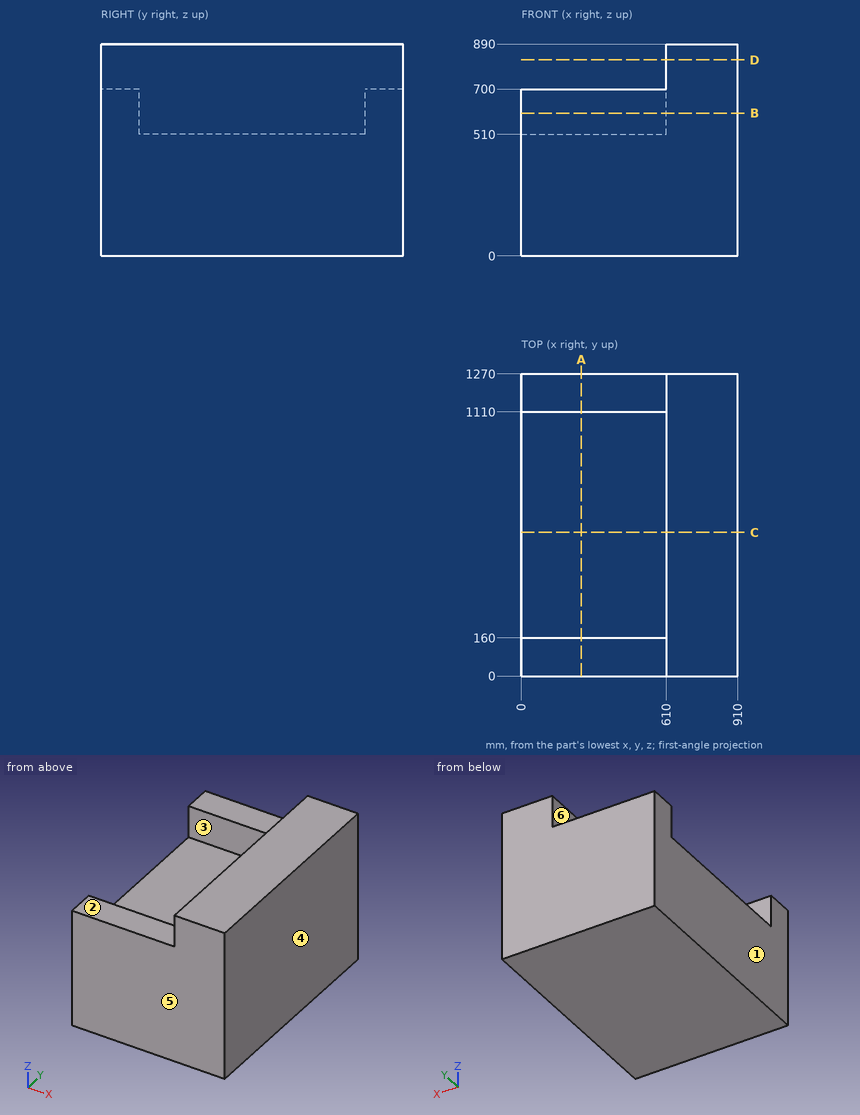
The figure shows three views and two pictorial views of one solid part (mm, origin at its lowest corner). Answer the questions. A direction names the side the tool comes from. Round coordinates to 2 decimals unless told otherwise and drop trailing zeros. Order: outer loops, then holes, each group sorted by start corner. A loop starts at its lowest first (then second) coordinate and runs counter-clockwise, first axis right, second up. Notation, with made-up numbers: (-13, -4.75) -> (14, -4.75) arc R10 cw to (14, -0.75) -> close; hole circle Ø7 at (82.5, 89). An arc over 180 degrees is marked (long way). One line per item, written item: value.
Item 1: Find section D-D, the plane z = 823. Give the vertices of the cut face in (x, y), then the cut area to 3 significant figures.
Taken from the geometry:
outline: (610, 0) -> (910, 0) -> (910, 1270) -> (610, 1270) -> close
area: 381,000 mm2
Item 2: For the marked faces 1, 2 and 3, determine the directions among +Z, -Z, +X, -X, +Y, -Y from which every point of the face is accessible in a straight line to the end or side of a thin tool.
Taken from the geometry:
face 1: +Z, -Z, -X, +Y, -Y
face 2: +Z, -X, +Y, -Y
face 3: +Z, -X
Item 3: Given P1, Ø10, axis at y = 164.5, z = 800.5, coming from the -X side, flat-ended and moving along its own axis, determine where the tip first touches the part or whether it passes through.
Taken from the geometry:
P1: stops at x = 610
Item 4: For a pull along Y with two mould halves and no side action, classify the marked faces 4, 5 and 6 as released by +Y, released by -Y, zero draft, split by the parting line, or undercut.
Taken from the geometry:
face 4: zero draft
face 5: released by -Y
face 6: undercut
Item 5: Find section A-A, the plane x = 252. Give the vertices of the cut face in (y, z), then the cut area to 4 significant figures.
Taken from the geometry:
outline: (0, 0) -> (1270, 0) -> (1270, 700) -> (1110, 700) -> (1110, 510) -> (160, 510) -> (160, 700) -> (0, 700) -> close
area: 708,500 mm2
Item 6: Straight lines are drawn through the part: L1, parallel to Y at x = 532, z = 691.5; L2, parallel to X at y = 509, z = 696.5; L3, parallel to Z at x = 547.5, y = 743. For each, find the intervals that lie inside material, in ascending order.
Taken from the geometry:
L1: y = 0 to 160, 1110 to 1270
L2: x = 610 to 910
L3: z = 0 to 510
Item 7: Find section B-B, the plane z = 600. Give the vertices of the cut face in (x, y), then the cut area to 3 significant figures.
Taken from the geometry:
outline: (0, 0) -> (910, 0) -> (910, 1270) -> (0, 1270) -> (0, 1110) -> (610, 1110) -> (610, 160) -> (0, 160) -> close
area: 576,000 mm2
Item 8: Find section C-C, the plane y = 604. Give the vertices of the cut face in (x, z), then the cut area to 3 significant figures.
Taken from the geometry:
outline: (0, 0) -> (910, 0) -> (910, 890) -> (610, 890) -> (610, 510) -> (0, 510) -> close
area: 578,000 mm2
